Solid Edge part; units mm, degrees
sketch "Sketch1" plane through (0, 0, 0) normal (0, -1, 0) x (1, 0, 0)
  line L0 (0, -12.5) -> (125, -12.4999)
  line L1 (0, 12.5) -> (125, 12.4999)
  arc A0 (125, -12.4999) -> (125, 12.4999) centre (125, 0) ccw
  arc A1 (0, 12.5) -> (0, -12.5) centre (0, 0) ccw
  circle A2 centre (125, 0) radius 6
  circle A3 centre (0, 0) radius 6
extrude "Protrusion1" add sketch "Sketch1" along normal mid plane 6
properties part number "7" material "Fe 410 W"
For this review, take the finished solid that the model builds, in its own axes (mm). Coordinates: 2 decimals unless noted, no trailing zeros. Loops run counter-clockwise (first coordinate to the right, second up) from the corner with the lowest first, then second, coordinate; pieces in that order, holes last. Notation, with made-up numbers: (56, 6.25) - (70, 6.25) arc R17 ccw to (70, 28.25) - close; hole circle Ø4 at (-23, 35). An arc over 180 degrees is marked (long way). Use one line per item in the form item = value. Start each with the question number.
1) To check wall thickness, follow probe 1 along Z at (x, y) = (125, -1.45); probe 2 along X at (y, z) = (1.25, 1); probe 3 along X at (y, z) = (1.8, 5.25). State the ranges of each line that lie inside material, in increasing order. Write a range as from..to.
2) Take a section at C-C (z = -9). State the section outline as (x, y) points.
3) Draft analysis for pull direction Z (two halves, no side actions). For faces 1 (the face through (62, 0, 12.5)), 2 (the face through (119, 0, 0)), 3 (the face through (137.497, 0.042, 0.275)), state which applies: released by +Z, released by -Z, zero draft, split by the parting line, or undercut.
4) Take a section at A-A (z = 0). State the section outline as (x, y) points.
5) For pin 1 (7 mm diameter, centred on x = 125, z = 0, fed in from +Y), flat-tipped, find the tip position at first contact; note if it passes through.
6) Take a section at B-B (y = 1.05). State the section outline as (x, z) points.
From the geometry:
q1.probe_1 = -12.5..-6, 6..12.5
q1.probe_2 = -12.46..-5.92, 5.92..119.08, 130.92..137.46
q1.probe_3 = -11.34..-2.9, 2.9..122.1, 127.9..136.34
q2.outline = (-8.67, -3) - (133.67, -3) - (133.67, 3) - (-8.67, 3) - close
q3.face_1 = released by +Z
q3.face_2 = undercut
q3.face_3 = split by the parting line
q4.outline = (-12.5, -3) - (-6, -3) - (-6, 3) - (-12.5, 3) - close; (6, -3) - (119, -3) - (119, 3) - (6, 3) - close; (131, -3) - (137.5, -3) - (137.5, 3) - (131, 3) - close
q5.pin_1 = through
q6.outline = (0, -12.5) - (125, -12.5) arc R12.5 ccw to (125, 12.5) - (0, 12.5) arc R12.5 ccw to start; hole circle Ø12 at (0, 0); hole circle Ø12 at (125, 0)
